```python
from build123d import *

# Parameters (mm, degrees)
BOSS_EXTRUDE1_DEPTH = 25
CUT_EXTRUDE1_DEPTH  = 112.208503688
CUT_EXTRUDE2_DEPTH  = 117.69747202
FILLET2_R           = 10


with BuildPart() as part:
    # Sketch1 → Boss-Extrude1 (new, symmetric)
    with BuildSketch(Plane.XY):
        Polygon((0, 0), (37.460659342, 92.718385457), (46.732497887, 88.972319523), (14.825609685, 10), (70, 10), (70, 0), align=None)
    extrude(amount=BOSS_EXTRUDE1_DEPTH, both=True)

    # Sketch2 → Cut-Extrude1 (cut, through all)
    with BuildSketch(Plane(origin=(0, 10, 0), x_dir=(1, 0, 0), z_dir=(0, 1, 0))):
        with BuildLine():
            Line((60, -3), (55, -3))
            ThreePointArc((55, -3), (52, 0), (55, 3))
            Line((55, 3), (60, 3))
            ThreePointArc((60, 3), (63, 0), (60, -3))
        make_face()
    extrude(amount=-CUT_EXTRUDE1_DEPTH, mode=Mode.SUBTRACT)

    # Sketch3 → Cut-Extrude2 (cut, through all)
    with BuildSketch(Plane(origin=(9.271838546, -3.746065934, 0), x_dir=(0, 0, -1), z_dir=(0.9271838545667856, -0.3746065934159163, 0))):
        with BuildLine():
            Line((3, 90), (3, 85))
            ThreePointArc((3, 85), (0, 82), (-3, 85))
            Line((-3, 85), (-3, 90))
            ThreePointArc((-3, 90), (0, 93), (3, 90))
        make_face()
    extrude(amount=-CUT_EXTRUDE2_DEPTH, mode=Mode.SUBTRACT)

    # Fillet2
    fillet2_edges = [part.edges().sort_by_distance(p)[0] for p in [
        (14.825609685, 10, 0),
    ]]
    fillet(fillet2_edges, radius=FILLET2_R)


solid = part.part
```
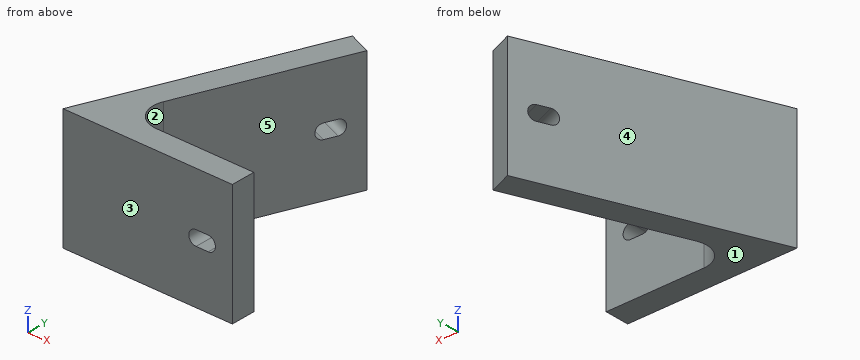
Part model, mm, in its own coordinate system. Face numbers are marked on the shaded views. A direction names the side the tool comes from. Coordinates: 2 decimals unless noted, no trailing zeros. Write each loop counter-clockwise with the first axis right and the second up, starting at its lowest first coordinate (ties: lowest second). Pieces come first, ordered by that corner, then holes.
Item 1: Slice it at A-A (x = 58.5). Write the cut outline in (y, z), and give its area (3 significant figures).
Item 2: Mould opens along Y. For the marked faces 1, 2 and 3 say: released by +Y, released by -Y, zero draft, split by the parting line, or undercut.
Item 3: Slice it at D-D (x = 45.5). Write the cut outline in (y, z), and give its area (3 significant figures).
Item 4: Which spindle directions (+Z, -Z, +X, -X, +Y, -Y) get a long thin tool onto all of the face, cutting with end or side? Do the marked faces 4 and 5. Say none if no direction does.
Item 5: Probe line 1 (Y direction, x = 25, z = -18); line 2 (Y direction, x = 35.5, z = -15.5); line 3 (Y direction, x = 58, z = -8.5). List the from-to ranges inside material, lowest first.
Item 6: Pin check, flat tips, straight feed: pin 1 (8 mm diameter, centred on y = 17, z = -11.5, fed in from -X); pin 2 (10 mm diameter, centred on x = 24, z = -16.5, fed in from +Y); pin 3 (4 mm diameter, centred on y = 14.5, z = 14.5, fed in from -X). Stop position of each tip, or through.
Item 7: Slice it at B-B (z = 0). Write the cut outline in (x, y), and give its area (3 significant figures).
Item 8: Slice it at C-C (z = -16.5). Write the cut outline in (x, y).
Results found:
1. outline: (0, -25) - (10, -25) - (10, -3) - (0, -3) - close; (0, 3) - (10, 3) - (10, 25) - (0, 25) - close
1. area: 440 mm2
2. face 1: zero draft
2. face 2: undercut
2. face 3: released by -Y
3. outline: (0, -25) - (10, -25) - (10, 25) - (0, 25) - close; (85.92, -25) - (89.47, -25) - (89.47, 25) - (85.92, 25) - close
3. area: 677 mm2
4. face 4: +Z, -Z, -X, +Y
4. face 5: +Z, -Z, +X
5. line 1: y = 0 to 11.15, 35.18 to 61.88
5. line 2: y = 0 to 10, 61.17 to 87.87
5. line 3: y = 0 to 10
6. pin 1: stops at x = 5.25
6. pin 2: stops at y = 71.78
6. pin 3: stops at x = 5.05
7. outline: (0, 0) - (52, 0) - (52, 10) - (29.65, 10) arc R10 cw to (20.38, 23.75) - (39.99, 72.28) - (30.72, 76.03) - close; (34.84, 86.23) - (44.11, 82.48) - (46.73, 88.97) - (37.46, 92.72) - close; (63, 0) - (70, 0) - (70, 10) - (63, 10) - close
7. area: 1,380 mm2
8. outline: (0, 0) - (70, 0) - (70, 10) - (29.65, 10) arc R10 cw to (20.38, 23.75) - (46.73, 88.97) - (37.46, 92.72) - close
